```python
from build123d import *

# Parameters (mm, degrees)
F1_DEPTH = 7.5
F2_R     = 50
F3_R     = 14.99999
F4_R     = 7.75
F5_DEPTH = 15


# Not quite as in the source:
# - a fillet or chamfer is up to 0.001 mm smaller than in the source, because OpenCascade refuses the exact size


with BuildPart() as f1:
    # F0 (on Front) → F1 (new body, symmetric)
    with BuildSketch(Plane.XZ):
        Polygon((92.5735931288, 0), (0, 0), (0, -30), (105, -30), (135, 0), (205, 0), (205, 30), (122.5735931288, 30), align=None)
    extrude(amount=F1_DEPTH, both=True)

    # F2
    f2_edges = [f1.edges().sort_by_distance(p)[0] for p in [
        (92.573593, 0, 0),
        (122.573593, 0, 30),
        (105, 0, -30),
        (135, 0, 0),
    ]]
    fillet(f2_edges, radius=F2_R)

    # F3 (radius 15 in the source; OpenCascade refuses exactly that, so slightly less here)
    f3_edges = [f1.edges().sort_by_distance(p)[0] for p in [
        (0, 0, 0),
        (0, 0, -30),
    ]]
    fillet(f3_edges, radius=F3_R)

    # F4 (on face) → F5 (cut, through all)
    with BuildSketch(Plane.XZ.offset(7.5)):
        with Locations((15, -15)):
            Circle(F4_R)
        with Locations((75, -15)):
            Circle(F4_R)
    extrude(amount=-F5_DEPTH, mode=Mode.SUBTRACT)


solid = f1.part
```
Geometry: final body of the model. Coordinates: model frame, mm. A direction names the side the tool comes from. Coordinates: 2 decimals unless noted, no trailing zeros. Order: outer loops, then holes, each group sorted by start corner. A loop starts at its lowest first (then second) coordinate and runs counter-clockwise, first axis right, second up. Notation, with made-up numbers: (17.25, 30) - (57.25, 30) arc R22 cw to (57.25, 54) - close; hole circle Ø1 at (-23.5, 86.25). An arc over 180 degrees is marked (long way). Return JSON: item names as keys, results as strings. Group by question number.
1. Set-up query: faces 5 (the face through (180, 0, 0)), 6 (the face through (175, 0, 30)). Return all of +Z, -Z, +X, -X, +Y, -Y with unobstructed straight access to the full face (end or side cutting, diameter ignored); none if empty.
2. Pin query (flat end, axial travel): pin 1 (7.5 mm diameter, centred on x = 169, y = -0.5, fed in from -Z); pin 2 (3 mm diameter, centred on y = 1.5, z = -19.5, fed in from -X); pin 3 (8 mm diameter, centred on y = -4, z = -18, fed in from +X). Return the tip coordinate at first contact, or that it passes through.
3. Cut plane B-B (x = 75). Output: boundary loops of the cut face in (y, z), plus the area to 3 significant figures.
4. Cut plane C-C (z = -21). Output: boundary loops of the cut face in (x, y).
5. Material intervals for line 1 along X through (y, z) = (-3.25, -14.5); line 2 along X through (y, z) = (6, -8); line 3 along Z through (x, y) = (15, 3.75), sorted ascending. Write a range as [from, to].
6. Cut plane A-A (y = 2). Count the separate pieces of the cut face and the enclosed holes in it, plus the area to 3 significant figures.
7. Pull-direction query (Z, two-part tool) for faces 1 (the face through (124, 7.5, 0)), 2 (the face through (103.677, -0.105, -26.088)), 3 (the face through (44, 0, 0)), 4 (the face through (22.16, -0.11, -17.97)); classes: pulls with the +Z half, pulls with the -Z half, needs draft (parallel to the pull), parting line crosses it, or undercut.
8. Cut plane D-D (x = 30). Output: boundary loops of the cut face in (y, z).
Resolved:
{
 "1": {"face 5": "-Z, +X, +Y, -Y", "face 6": "+Z, +X, -X, +Y, -Y"},
 "2": {"pin 1": "stops at z = 0", "pin 2": "stops at x = 0.3", "pin 3": "stops at x = 121.01"},
 "3": {"outline": "(-7.5, -30) - (7.5, -30) - (7.5, -22.75) - (-7.5, -22.75) - close; (-7.5, -7.25) - (7.5, -7.25) - (7.5, 0.1) - (-7.5, 0.1) - close", "area": "219 mm²"},
 "4": {"outline": "(1.25, -7.5) - (10.09, -7.5) - (10.09, 7.5) - (1.25, 7.5) - close; (19.91, -7.5) - (70.09, -7.5) - (70.09, 7.5) - (19.91, 7.5) - close; (79.91, -7.5) - (112.91, -7.5) - (112.91, 7.5) - (79.91, 7.5) - close"},
 "5": {"line 1": "x = [0.01, 7.27], [22.73, 67.27], [82.73, 120.5]", "line 2": "x = [1.73, 11.67], [18.33, 71.67], [78.33, 128.58]", "line 3": "z = [-30, -22.75], [-7.25, 0]"},
 "6": {"separate pieces": "1", "enclosed holes": "2", "area": "6,050 mm²"},
 "7": {"face 1": "needs draft", "face 2": "pulls with the -Z half", "face 3": "pulls with the +Z half", "face 4": "undercut"},
 "8": {"outline": "(-7.5, -30) - (7.5, -30) - (7.5, 0) - (-7.5, 0) - close"}
}
